Answer from the drawing. Dimensions are ordinates in mm from the lowest x, y and z of the part. A direction names the side the tool comes from. Give positions to 0.01 mm unless a question says otherwise; leave off trailing zeros. Write each loop counter-clockwise with the first axis right and the second up, starting at its lowest first coordinate (ties: lowest second). Pieces come first, ordered by that corner, then holes. Notation, with made-up numbers: M 72,83.5 L 105,83.5 A33 ccw 105,121.5 Z; hole C -17,60.25 d10. An arc over 180 degrees is marked long. Write each question's results on one line, items separated by ' | '. Start each with the question number.
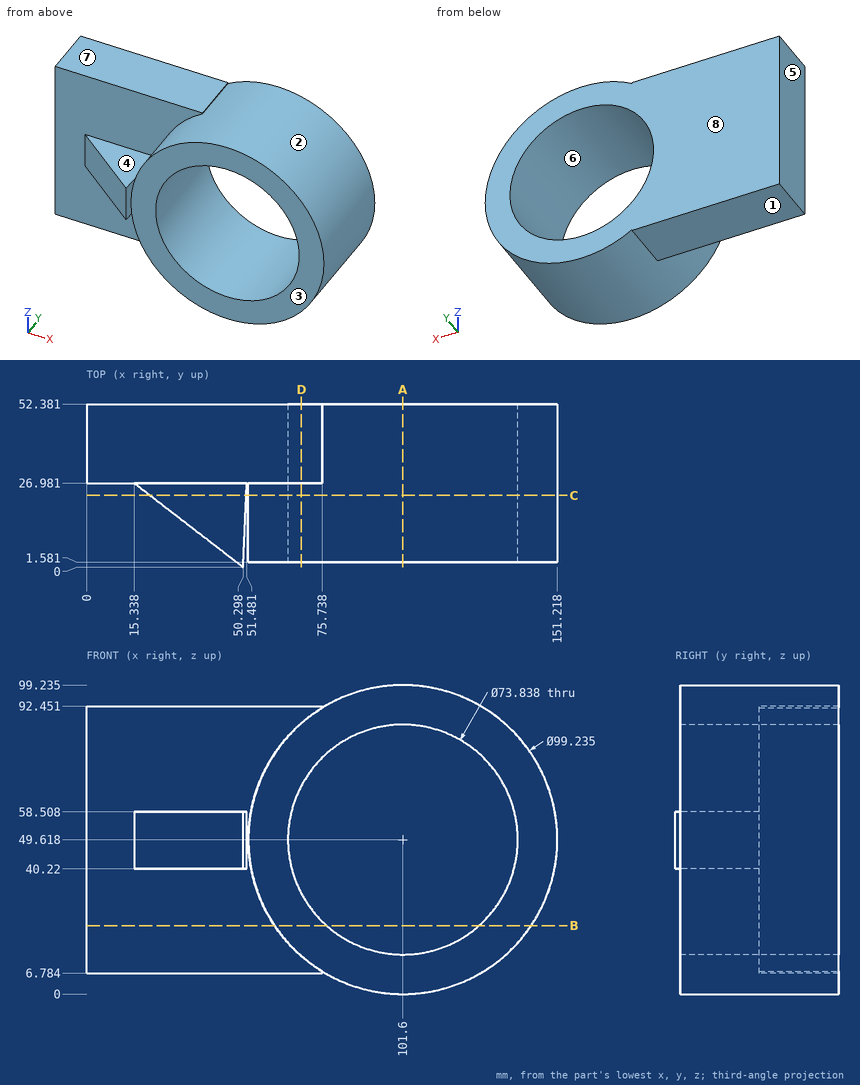
Item 1: Determine the mould class of the marked faces 6, 7 and 8 for opening direction Z: +Z half, -Z half, draft (parallel to the pull), parting line (faces both ways), or undercut.
Item 2: Section A-A, the plane x = 101.6 is taken. Determine the outline of the cut face in (y, z) (1 decimal), then the cut area to 3 significant figures.
Item 3: For the marked faces 1, 2, 3, 4 and 5, determine the directions among +Z, -Z, +X, -X, +Y, -Y from which every point of the face is accessible in a straight line to the end or side of a thin tool.
Item 4: Given P1, Ø5, axis at x = 68, y = 10.5, coming from the -Z side (1 decimal); P2, Ø2, axis at y = 22, z = 83.5, coming from the +X side; P3, Ø1, axis at x = 133.5, z = 88, coming from the +Y side; P4, Ø20.5, axis at x = 49, y = 44.5, coming from the -Z side, each flat-ended and moving along its own axis, determine where each tip first touches the part or whether it passes through.
Item 5: Section D-D, the plane x = 69 is taken. Determine the outline of the cut face in (y, z) (1 decimal), then the cut area to 3 significant figures.
Item 6: Section B-B, the plane z = 22 is taken. Determine the outline of the cut face in (x, y).
Item 7: Section C-C, the plane y = 23 is taken. Determine the outline of the cut face in (x, z) (1 decimal), then the cut area to 3 significant figures.
Item 8: Straight lines are drawn through the part: line 1 (Z direction, x = 101, y = 15); line 2 (Y direction, x = 70.5, z = 22.5); line 3 (X direction, y = 21, z = 54.5) (1 decimal). For each, find the intervals that lie inside material, in ascending order.
Worked out:
1) face 6: undercut | face 7: +Z half | face 8: draft
2) outline: M 1.6,0 L 52.4,0 L 52.4,12.7 L 1.6,12.7 Z; M 1.6,86.5 L 52.4,86.5 L 52.4,99.2 L 1.6,99.2 Z | area: 1,290 mm²
3) face 1: -Z, -X, +Y, -Y | face 2: -Y | face 3: +Z, -Z, +X, -Y | face 4: +Z, -X, -Y | face 5: +Z, -Z, -X, +Y, -Y
4) P1: stops at z = 11 | P2: stops at x = 138.76 | P3: stops at y = 52.38 | P4: stops at z = 6.78
5) outline: M 1.6,12.2 L 27,12.2 L 27,6.8 L 52.4,6.8 L 52.4,32.3 L 1.6,32.3 Z; M 1.6,66.9 L 52.4,66.9 L 52.4,92.5 L 27,92.5 L 27,87 L 1.6,87 Z | area: 2,320 mm²
6) outline: M 0,26.98 L 60.38,26.98 L 60.38,1.58 L 77.1,1.58 L 77.1,52.38 L 0,52.38 Z; M 126.1,1.58 L 142.82,1.58 L 142.82,52.38 L 126.1,52.38 Z
7) outline: M 20.5,40.2 L 51.3,40.2 L 51.3,58.5 L 20.5,58.5 Z; C 101.6,49.6 d99.2; hole C 101.6,49.6 d73.8 | area: 4,020 mm²
8) line 1: z = 0 to 12.7, 86.53 to 99.23 | line 2: y = 1.58 to 52.38 | line 3: x = 23.1 to 51.2, 52.2 to 65, 138.2 to 151
